from build123d import *

# Parameters (mm, degrees)
F1_DEPTH = 44.45
F2_DEPTH = 38.1
F3_DEPTH = 8.92661


with BuildPart() as f1:
    # F0 (on Top) → F1 (new body)
    with BuildSketch(Plane.XY):
        Polygon((59.9326238802, -10.0844367775), (59.9326238802, 30.48), (47.2326238802, 30.48), (47.2326238802, 38.1), (34.5326238802, 38.1), (34.5326238802, 47.8773999231), (9.1326238802, 47.8773999231), (4.5917662157, 47.8773999231), (-5.5682337843, 47.8773999231), (-10.1090914488, 47.8773999231), (-35.5090914488, 47.8773999231), (-35.5090914488, 38.1), (-48.2090914488, 38.1), (-48.2090914488, 30.48), (-60.9090914488, 30.48), (-60.9090914488, -10.16), (-52.4551342213, -10.16), (-37.2151342213, -10.16), (-37.2151342213, -4.8143821768), (33.9048657787, -4.8143821768), (33.9048657787, -10.16), (49.1448657787, -10.16), align=None)
        Polygon((-58.2453422248, 12.9522867501), (-58.2453422248, 21.7635072768), (-46.8229997575, 21.7635072768), (-46.8229997575, 31.4483940601), (-34.1229997575, 31.4483940601), (-34.1229997575, 42.2507673502), (-21.4229997575, 42.2507673502), (19.4527748972, 42.2507673502), (32.1527748972, 42.2507673502), (32.1527748972, 31.4483940601), (45.6809252501, 31.4483940601), (45.6809252501, 21.018518135), (56.1551556194, 21.018518135), (56.1551556194, 12.9522867501), (56.1551556194, 0), (56.1551556194, -7.2993603218), (38.3249066973, -7.2993603218), (38.3249066973, -0.0041214007), (-40.4150933027, -0.0041214007), (-40.4150933027, -8.0205244012), (-58.2453422248, -8.0205244012), (-58.2453422248, 0), align=None, mode=Mode.SUBTRACT)
        Polygon((49.1448657787, -29.6408813447), (49.1448657787, -10.16), (33.9048657787, -10.16), (33.9048657787, -4.8143821768), (-37.2151342213, -4.8143821768), (-37.2151342213, -10.16), (-52.4551342213, -10.16), (-52.4551342213, -29.6408813447), (-39.7551342213, -29.6408813447), (-39.7551342213, -38.5807752609), (-33.4051342213, -38.5807752609), (-33.4051342213, -45.2856980264), (30.0948657787, -45.2856980264), (30.0948657787, -38.5807752609), (36.4448657787, -38.5807752609), (36.4448657787, -29.6408813447), align=None)
        Polygon((31.5474388957, -16.645764932), (44.2474388957, -16.645764932), (44.2474388957, -26.2884218246), (31.5474388957, -26.2884218246), (31.5474388957, -32.2483479977), (25.1974388957, -32.2483479977), (25.1974388957, -41.1882456392), (-28.3929689348, -41.1882456392), (-28.3929689348, -34.483326599), (-34.7429689348, -34.483326599), (-34.7429689348, -26.2884218246), (-47.4429689348, -26.2884218246), (-47.4429689348, -16.645764932), (-34.7429689348, -16.645764932), (-34.7429689348, -7.755764932), (-20.0950933027, -7.755764932), (-15.0150933027, -7.755764932), (12.9249066973, -7.755764932), (18.0049066973, -7.755764932), (31.5474388957, -7.755764932), align=None, mode=Mode.SUBTRACT)
        Polygon((-46.8229997575, 21.7635072768), (-58.2453422248, 21.7635072768), (-58.2453422248, 12.9522867501), (-50.0864312053, 12.9522867501), (-50.0864312053, 19.0039230511), (-43.8020415604, 19.0039230511), (-43.8020415604, 3.4093181603), (-50.0864312053, 3.4093181603), (-50.0864312053, 0), (-58.2453422248, 0), (-58.2453422248, -8.0205244012), (-40.4150933027, -8.0205244012), (-40.4150933027, -0.0041214007), (38.3249066973, -0.0041214007), (38.3249066973, -7.2993603218), (56.1551556194, -7.2993603218), (56.1551556194, 0), (51.3948649168, 0), (51.3948649168, 3.4093209542), (41.711854955, 3.4093209542), (41.711854955, 15.5125940219), (50.4638440907, 15.5125940219), (50.4638440907, 12.9522867501), (56.1551556194, 12.9522867501), (56.1551556194, 21.018518135), (45.6809252501, 21.018518135), (32.1527748972, 21.018518135), (32.1527748972, 25.9544569999), (25.0515304506, 25.9544569999), (25.0515304506, 31.4483940601), (19.4527748972, 31.4483940601), (19.4527748972, 42.2507673502), (-21.4229997575, 42.2507673502), (-21.4229997575, 31.4483940601), (-27.7042705566, 31.4483940601), (-27.7042705566, 26.4783278108), (-34.1229997575, 26.4783278108), (-34.1229997575, 21.7635072768), align=None)
        Polygon((18.0049066973, 0), (-20.0950933027, 0), (-20.0950933027, 3.511225339), (-24.4833528996, 3.511225339), (-24.4833528996, 19.0039230511), (-20.0950933027, 19.0039230511), (-20.0950933027, 24.1245422512), (18.0049066973, 24.1245422512), (18.0049066973, 19.702189602), (22.3931662941, 19.702189602), (22.3931662941, 4.2094918899), (18.0049066973, 4.2094918899), align=None, mode=Mode.SUBTRACT)
        Polygon((44.2474388957, -26.2884218246), (44.2474388957, -16.645764932), (31.5474388957, -16.645764932), (31.5474388957, -7.755764932), (18.0049066973, -7.755764932), (18.0049066973, -20.455764932), (12.9249066973, -20.455764932), (12.9249066973, -7.755764932), (-15.0150933027, -7.755764932), (-15.0150933027, -20.455764932), (-20.0950933027, -20.455764932), (-20.0950933027, -7.755764932), (-34.7429689348, -7.755764932), (-34.7429689348, -16.645764932), (-47.4429689348, -16.645764932), (-47.4429689348, -26.2884218246), (-34.7429689348, -26.2884218246), (-34.7429689348, -34.483326599), (-28.3929689348, -34.483326599), (-28.3929689348, -41.1882456392), (25.1974388957, -41.1882456392), (25.1974388957, -32.2483479977), (31.5474388957, -32.2483479977), (31.5474388957, -26.2884218246), align=None)
        Polygon((4.5917662157, 47.8773999231), (9.1326238802, 47.8773999231), (9.1326238802, 60.5773999231), (-10.1090914488, 60.5773999231), (-10.1090914488, 47.8773999231), (-5.5682337843, 47.8773999231), (-5.5682337843, 55.2843213081), (4.5917662157, 55.2843213081), align=None)
    extrude(amount=-F1_DEPTH)

    # F0 (on Top) → F2 (join)
    with BuildSketch(Plane.XY):
        Polygon((32.1527748972, 42.2507673502), (19.4527748972, 42.2507673502), (19.4527748972, 31.4483940601), (25.0515304506, 31.4483940601), (25.0515304506, 25.9544569999), (32.1527748972, 25.9544569999), (32.1527748972, 21.018518135), (45.6809252501, 21.018518135), (45.6809252501, 31.4483940601), (32.1527748972, 31.4483940601), align=None)
        Polygon((51.3948649168, 0), (56.1551556194, 0), (56.1551556194, 12.9522867501), (50.4638440907, 12.9522867501), (50.4638440907, 15.5125940219), (41.711854955, 15.5125940219), (41.711854955, 3.4093209542), (51.3948649168, 3.4093209542), align=None)
        Polygon((-20.0950933027, 3.511225339), (-20.0950933027, 0), (18.0049066973, 0), (18.0049066973, 4.2094918899), (22.3931662941, 4.2094918899), (22.3931662941, 19.702189602), (18.0049066973, 19.702189602), (18.0049066973, 24.1245422512), (-20.0950933027, 24.1245422512), (-20.0950933027, 19.0039230511), (-24.4833528996, 19.0039230511), (-24.4833528996, 3.511225339), align=None)
        Polygon((-46.8229997575, 31.4483940601), (-46.8229997575, 21.7635072768), (-34.1229997575, 21.7635072768), (-34.1229997575, 26.4783278108), (-27.7042705566, 26.4783278108), (-27.7042705566, 31.4483940601), (-21.4229997575, 31.4483940601), (-21.4229997575, 42.2507673502), (-34.1229997575, 42.2507673502), (-34.1229997575, 31.4483940601), align=None)
        Polygon((-50.0864312053, 12.9522867501), (-58.2453422248, 12.9522867501), (-58.2453422248, 0), (-50.0864312053, 0), (-50.0864312053, 3.4093181603), (-43.8020415604, 3.4093181603), (-43.8020415604, 19.0039230511), (-50.0864312053, 19.0039230511), align=None)
    extrude(amount=-F2_DEPTH)

    # F0 (on Top) → F3 (cut)
    with BuildSketch(Plane.XY):
        Polygon((-50.0864312053, 12.9522867501), (-58.2453422248, 12.9522867501), (-58.2453422248, 0), (-50.0864312053, 0), (-50.0864312053, 3.4093181603), (-43.8020415604, 3.4093181603), (-43.8020415604, 19.0039230511), (-50.0864312053, 19.0039230511), align=None)
        Polygon((-46.8229997575, 31.4483940601), (-46.8229997575, 21.7635072768), (-34.1229997575, 21.7635072768), (-34.1229997575, 26.4783278108), (-27.7042705566, 26.4783278108), (-27.7042705566, 31.4483940601), (-21.4229997575, 31.4483940601), (-21.4229997575, 42.2507673502), (-34.1229997575, 42.2507673502), (-34.1229997575, 31.4483940601), align=None)
        Polygon((-20.0950933027, 3.511225339), (-20.0950933027, 0), (18.0049066973, 0), (18.0049066973, 4.2094918899), (22.3931662941, 4.2094918899), (22.3931662941, 19.702189602), (18.0049066973, 19.702189602), (18.0049066973, 24.1245422512), (-20.0950933027, 24.1245422512), (-20.0950933027, 19.0039230511), (-24.4833528996, 19.0039230511), (-24.4833528996, 3.511225339), align=None)
        Polygon((32.1527748972, 42.2507673502), (19.4527748972, 42.2507673502), (19.4527748972, 31.4483940601), (25.0515304506, 31.4483940601), (25.0515304506, 25.9544569999), (32.1527748972, 25.9544569999), (32.1527748972, 21.018518135), (45.6809252501, 21.018518135), (45.6809252501, 31.4483940601), (32.1527748972, 31.4483940601), align=None)
        Polygon((51.3948649168, 0), (56.1551556194, 0), (56.1551556194, 12.9522867501), (50.4638440907, 12.9522867501), (50.4638440907, 15.5125940219), (41.711854955, 15.5125940219), (41.711854955, 3.4093209542), (51.3948649168, 3.4093209542), align=None)
    extrude(amount=-F3_DEPTH, mode=Mode.SUBTRACT)


solid = f1.part
Source: CAD feature listing. Evaluate the final solid. Frame: model axes, mm. A direction names the side the tool comes from. Coordinates: 2 decimals unless noted, no trailing zeros. Loops run counter-clockwise (first coordinate to the right, second up) from the corner with the lowest first, then second, coordinate; pieces in that order, holes last. Notation, with made-up numbers: (88, 25) -> (145, 25) arc R15 ccw to (145, 47) -> close; hole circle Ø9 at (-27.5, 68). An arc over 180 degrees is marked (long way). Answer in a Markdown table with one row per item. Add a question column.
Q1. Reachability of faces 1 (the face through (-47, 19.004, -4)), 2 (the face through (22, 31.448, -41)), 3 (the face through (-1, -3, 0)) from +Z, -Z, +X, -X, +Y, -Y: full face, straight path, thin tool, end or side. Return the list, or none.
Q2. Ray query, line 1 along X through (y, z) = (14.5, -5); line 2 along X through (y, z) = (37.5, -4.5); line 3 along X through (y, z) = (-12.5, -25). Return the intervals inside material, ascending.
Q3. Section A-A on x = 16.5. Return the cut outline in (y, z), and give its area (3 significant figures).
Q4. Pull-direction query (X, two-part tool) for faces 4 (the face through (34.533, 43, -22)), 5 (the face through (-57, -10.16, -22)), 6 (the face through (41.712, 9, -41)); classes: pulls with the +X half, pulls with the -X half, needs draft (parallel to the pull), parting line crosses it, or undercut.
Q5. Section C-C on z = -39.5. Give the number of separate pieces and of enclosed holes in the cut face, and give its area (3 significant figures).
Q6. Section D-D on x = -38. Return the cut outline in (y, z).
Q7. Section B-B on y = 33. Return the cut outline in (x, z).
Q8. Contact query for flat-ended pins moving along their axis: pin 1 Ø3 at (y, z) = (-18, -18) entering from +X; pin 2 Ø3.5 at (x, z) = (-21.5, -40.5) entering from +Y; pin 3 Ø8 at (y, z) = (40, -33) entering from +X. Output: stop coordinate, or through.
Computed values:
| question | item | result |
|---|---|---|
| 1 | face 1 | +Z |
| 1 | face 2 | -Z |
| 1 | face 3 | +Z, +X, -X, +Y, -Y |
| 2 | line 1 | x = -60.91 to -50.09, -43.8 to -24.48, 22.39 to 41.71, 50.46 to 59.93 |
| 2 | line 2 | x = -48.21 to -34.12, -21.42 to 19.45, 32.15 to 47.23 |
| 2 | line 3 | x = -52.46 to -20.1, -15.02 to 12.92, 18 to 49.14 |
| 3 | outline | (-45.29, -44.45) -> (-20.46, -44.45) -> (-20.46, 0) -> (-45.29, 0) -> close; (-7.76, -44.45) -> (0, -44.45) -> (0, -38.1) -> (24.12, -38.1) -> (24.12, -44.45) -> (47.88, -44.45) -> (47.88, 0) -> (24.12, 0) -> (24.12, -8.93) -> (0, -8.93) -> (0, 0) -> (-7.76, 0) -> close |
| 3 | area | 3,210 mm^2 |
| 4 | face 4 | pulls with the +X half |
| 4 | face 5 | needs draft |
| 4 | face 6 | undercut |
| 5 | separate pieces | 1 |
| 5 | enclosed holes | 8 |
| 5 | area | 7,400 mm^2 |
| 6 | outline | (-38.58, -44.45) -> (21.76, -44.45) -> (21.76, -38.1) -> (31.45, -38.1) -> (31.45, -44.45) -> (38.1, -44.45) -> (38.1, 0) -> (31.45, 0) -> (31.45, -8.93) -> (21.76, -8.93) -> (21.76, 0) -> (-38.58, 0) -> close |
| 7 | outline | (-48.21, -44.45) -> (-34.12, -44.45) -> (-34.12, -38.1) -> (-21.42, -38.1) -> (-21.42, -44.45) -> (19.45, -44.45) -> (19.45, -38.1) -> (32.15, -38.1) -> (32.15, -44.45) -> (47.23, -44.45) -> (47.23, 0) -> (32.15, 0) -> (32.15, -8.93) -> (19.45, -8.93) -> (19.45, 0) -> (-21.42, 0) -> (-21.42, -8.93) -> (-34.12, -8.93) -> (-34.12, 0) -> (-48.21, 0) -> close |
| 8 | pin 1 | stops at x = 49.14 |
| 8 | pin 2 | stops at y = 47.88 |
| 8 | pin 3 | stops at x = 47.23 |
